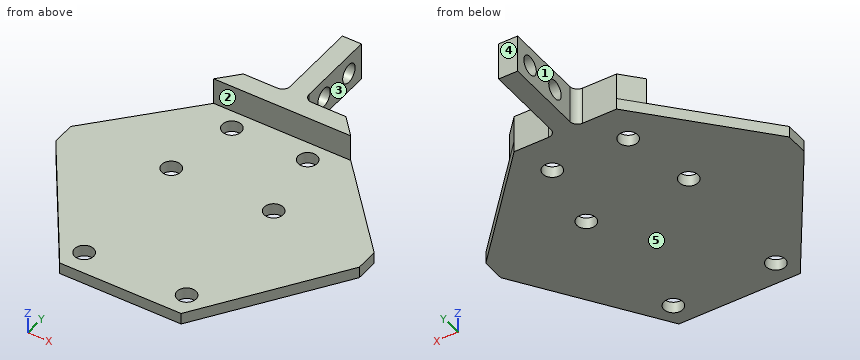
from build123d import *

# Parameters (mm, degrees)
SKETCH2_R                = 2.5
BOSS_EXTRUDE1_DEPTH      = 3
BOSS_EXTRUDE2_DEPTH      = 7
BOSS_EXTRUDE4_DEPTH      = 2.8
BOSS_EXTRUDE4_DEPTH_BACK = 2.2
SKETCH7_W                = 10
SKETCH7_H                = 23
SKETCH7_R                = 2.5
SKETCH9_R                = 2.5
CUT_EXTRUDE1_DEPTH       = 10
FILLET5_R                = 2


with BuildPart() as part:
    # Sketch2 → Boss-Extrude1 (new body)
    with BuildSketch(Plane.XY):
        Polygon((16, -41), (40, -6), (40, 0), (13.5, 29), (-13.5, 29), (-40, 0), (-40, -6), (-16, -41), align=None)
        with Locations((-13.5, 0)):
            Circle(SKETCH2_R, mode=Mode.SUBTRACT)
        with Locations((13.5, 0)):
            Circle(SKETCH2_R, mode=Mode.SUBTRACT)
        with Locations((13.5, -35)):
            Circle(SKETCH2_R, mode=Mode.SUBTRACT)
        with Locations((-13.5, -35)):
            Circle(SKETCH2_R, mode=Mode.SUBTRACT)
    extrude(amount=BOSS_EXTRUDE1_DEPTH)

    # Sketch4 → Boss-Extrude2 (add)
    with BuildSketch(Plane.XY.offset(3)):
        Polygon((-13.5, 29), (-18.068965517, 24), (18.068965517, 24), (13.5, 29), align=None)
    extrude(amount=BOSS_EXTRUDE2_DEPTH)

    # Sketch7 → Boss-Extrude4 (add, two sides: drawn at the far end of the back side and taken through both)
    with BuildSketch(Plane(origin=(-0.30437935, -56.168103165, -48.676228962), x_dir=(0, 0, -1), z_dir=(1, 0, 0)).offset(-BOSS_EXTRUDE4_DEPTH_BACK)):
        with Locations((-53.676228962, 96.668103165)):
            Rectangle(SKETCH7_W, SKETCH7_H)
        with Locations((-53.676228962, 103.168103165)):
            Circle(SKETCH7_R, mode=Mode.SUBTRACT)
        with Locations((-53.676228962, 93.168103165)):
            Circle(SKETCH7_R, mode=Mode.SUBTRACT)
    extrude(amount=BOSS_EXTRUDE4_DEPTH + BOSS_EXTRUDE4_DEPTH_BACK)

    # Sketch9 → Cut-Extrude1 (cut)
    with BuildSketch(Plane.XY.offset(3)):
        with Locations((-10, 19)):
            Circle(SKETCH9_R)
        with Locations((10, 19)):
            Circle(SKETCH9_R)
    extrude(amount=-CUT_EXTRUDE1_DEPTH, mode=Mode.SUBTRACT)

    # Fillet5
    fillet5_edges = [part.edges().sort_by_distance(p)[0] for p in [
        (-2.50437935, 29, 5),
        (2.49562065, 29, 5),
    ]]
    fillet(fillet5_edges, radius=FILLET5_R)


solid = part.part
Input: part model. Units: mm. Frame: model coordinates. Face numbers are marked on the shaded views. A direction names the side the tool comes from. Coordinates: 2 decimals unless noted, no trailing zeros. Order: outer loops, then holes, each group sorted by start corner. A loop starts at its lowest first (then second) coordinate and runs counter-clockwise, first axis right, second up. Notation, with made-up numbers: M 18.5,89 L 49.5,89 A14 cw 49.5,116 Z; hole C 59.5,52 d7. An arc over 180 degrees is marked long. Answer in a Markdown table with one row per item.
(1) Contact query for flat-ended pins moving along their axis: pin 1 Ø5 at (y, z) = (44, 4) entering from -X; pin 2 Ø12 at (x, y) = (-10.5, -5) entering from +Z; pin 3 Ø3.5 at (x, z) = (8, 7.5) entering from -Y. Output: stop coordinate, or through.
Numbers:
| item | result |
|---|---|
| pin 1 | stops at x = -2.5 |
| pin 2 | stops at z = 3 |
| pin 3 | stops at y = 24 |
(2) Material intervals for line 1 (Y direction, x = -13.5, z = 1.55); line 2 (Z direction, x = -23.5, y = 8); line 3 (X direction, y = 40, z = 7.25), sorted ascending. Write a range as [from, to].
Numbers:
| item | result |
|---|---|
| line 1 | y = [-41, -37.5], [-32.5, -2.5], [2.5, 29] |
| line 2 | z = [0, 3] |
| line 3 | x = [-2.5, 2.5] |
(3) Access query for the marked faces 1, 2, 3, 4 and 5. Directions: +Z, -Z, +X, -X, +Y, -Y. A direction counts if a zero-diameter tool reaches every point of the face in a straight line with its end or side. Return the directions, or none.
Numbers:
| item | result |
|---|---|
| face 1 | +Z, -Z, -X, +Y |
| face 2 | +Z, +X, -X, -Y |
| face 3 | +Z, -Z, +X, +Y |
| face 4 | +Z, -Z, +X, -X, +Y |
| face 5 | -Z, +X, -X, +Y, -Y |
(4) Section query A-A, the plane z = 5. Output: boundary loops of the cut face in (x, y), plus the area to 3 significant figures.
Numbers:
| item | result |
|---|---|
| outline | M -18.07,24 L 18.07,24 L 13.5,29 L 4.5,29 A2 cw 2.5,31 L 2.5,34.5 L -2.5,34.5 L -2.5,31 A2 cw -4.5,29 L -13.5,29 Z; M -2.5,39.5 L 2.5,39.5 L 2.5,44.5 L -2.5,44.5 Z; M -2.5,49.5 L 2.5,49.5 L 2.5,52 L -2.5,52 Z |
| area | 225 mm^2 |
(5) Section query C-C, the plane y = 19. Output: boundary loops of the cut face in (x, z), plus the area to 3 significant figures.
Numbers:
| item | result |
|---|---|
| outline | M -22.64,0 L -12.5,0 L -12.5,3 L -22.64,3 Z; M -7.5,0 L 7.5,0 L 7.5,3 L -7.5,3 Z; M 12.5,0 L 22.64,0 L 22.64,3 L 12.5,3 Z |
| area | 106 mm^2 |
(6) Section query B-B, the plane x = -10. Output: boundary loops of the cut face in (y, z), plus the area to 3 significant figures.
Numbers:
| item | result |
|---|---|
| outline | M -41,0 L 16.5,0 L 16.5,3 L -41,3 Z; M 21.5,0 L 29,0 L 29,10 L 24,10 L 24,3 L 21.5,3 Z |
| area | 230 mm^2 |
(7) Section query D-D, the plane y = -18. Output: boundary loops of the cut face in (x, z).
Numbers:
| item | result |
|---|---|
| outline | M -31.77,0 L 31.77,0 L 31.77,3 L -31.77,3 Z |
